Design review of the part built by this model. Coordinates are the model's own, in mm. A direction names the side the tool comes from. Give positions to 0.01 mm unless a question says otherwise; leave off trailing zeros. Loops run counter-clockwise (first coordinate to the right, second up) from the corner with the lowest first, then second, coordinate; pieces in that order, holes last. Notation, with made-up numbers: (7, 59) -> (35, 59) arc R20 cw to (35, 79) -> close; hole circle Ø3 at (24.5, 27). An arc over 180 degrees is marked (long way). Use a Markdown table: item, result. Add a question column.
1. For pin 1 Ø6 at (y, z) = (-5, 3) entering from -X; pin 2 Ø1.5 at (x, y) = (9, -1) entering from -Z; pin 3 Ø1.8 at (x, y) = (5.5, 18.5) entering from +Z; pin 4 Ø3 at (x, y) = (9, 17) entering from -Z, all flat-tipped, find the tip position at first contact; note any pin that passes through.
2. Add section D-D (z = 19). State the section outline as (x, y) points.
3. Draft analysis for pull direction X (two halves, no side actions). For faces 1 (the flat face through (0, 0, 14)), 2 (the flat face through (8, -16, 25)), 3 (the flat face through (5, -23, 32)), state which applies: pulls with the +X half, pulls with the -X half, needs draft (parallel to the pull), parting line crosses it, or undercut.
4. Add section B-B (z = 5.5). State the section outline as (x, y) points.
5. For faces 4 (the cylindrical face through (5, 0, -14)), 5 (the flat face through (5, 21, 25)), list the 3-axis set-ups (+Z, -Z, +X, -X, +Y, -Y) from which the entire face can be reached by the end or side of a thin tool; tool diameter is ignored.
6. To check wall thickness, follow line 1 (Z direction, x = 4.25, y = 0); line 2 (Y direction, x = 6.75, z = 26.5); line 3 (X direction, y = -16, z = 29.5). State the ranges of each line that lie inside material, in increasing order.
7. Add section C-C (y = -15). State the section outline as (x, z) points.
8. Add section A-A (y = 0). State the section outline as (x, z) points, and give its area (3 significant figures).
```python
from build123d import *

# Parameters (mm, degrees)
F0_R     = 10
F1_DEPTH = 10
F2_R     = 1
F3_R     = 2
F4_W     = 6
F4_H     = 10
F5_DEPTH = 15
F6_R     = 2


with BuildPart() as f1:
    # F0 (on Right) → F1 (new body)
    with BuildSketch(Plane.YZ):
        with BuildLine():
            Line((24, 32), (-24, 32))
            Line((-24, 32), (-24, 18))
            Line((-24, 18), (-14, 0))
            ThreePointArc((-14, 0), (0, -14), (14, 0))
            Line((14, 0), (24, 18))
            Line((24, 18), (24, 32))
        make_face()
        Circle(F0_R, mode=Mode.SUBTRACT)
    extrude(amount=F1_DEPTH)

    # F2
    f2_edges = [f1.edges().sort_by_distance(p)[0] for p in [
        (0, 0, -14),
        (10, 0, -14),
    ]]
    fillet(f2_edges, radius=F2_R)

    # F3
    f3_edges = [f1.edges().sort_by_distance(p)[0] for p in [
        (0, 0, 32),
        (10, 0, 32),
    ]]
    fillet(f3_edges, radius=F3_R)

    # F4 (on face) → F5 (cut)
    with BuildSketch(Plane.XY.offset(32)):
        with Locations((5, 16)):
            Rectangle(F4_W, F4_H)
        with Locations((5, -16)):
            Rectangle(F4_W, F4_H)
    extrude(amount=-F5_DEPTH, mode=Mode.SUBTRACT)

    # F6
    f6_edges = [f1.edges().sort_by_distance(p)[0] for p in [
        (2, 21, 24.5),
        (8, 21, 24.5),
        (8, 11, 24.5),
        (2, 11, 24.5),
        (2, -21, 24.5),
        (8, -21, 24.5),
        (8, -11, 24.5),
        (2, -11, 24.5),
    ]]
    fillet(f6_edges, radius=F6_R)


solid = f1.part
```
Taken from the geometry:
| question | item | result |
|---|---|---|
| 1 | pin 1 | passes through |
| 1 | pin 2 | stops at z = -14 |
| 1 | pin 3 | stops at z = 17 |
| 1 | pin 4 | stops at z = 2.7 |
| 2 | outline | (0, -24) -> (10, -24) -> (10, 24) -> (0, 24) -> close; hole (2, -19) arc R2 ccw to (4, -21) -> (6, -21) arc R2 ccw to (8, -19) -> (8, -13) arc R2 ccw to (6, -11) -> (4, -11) arc R2 ccw to (2, -13) -> close; hole (2, 13) arc R2 ccw to (4, 11) -> (6, 11) arc R2 ccw to (8, 13) -> (8, 19) arc R2 ccw to (6, 21) -> (4, 21) arc R2 ccw to (2, 19) -> close |
| 3 | face 1 | pulls with the -X half |
| 3 | face 2 | undercut |
| 3 | face 3 | needs draft |
| 4 | outline | (0, -17.06) -> (10, -17.06) -> (10, -8.35) -> (0, -8.35) -> close; (0, 8.35) -> (10, 8.35) -> (10, 17.06) -> (0, 17.06) -> close |
| 5 | face 4 | -Z, +X, -X |
| 5 | face 5 | +Z |
| 6 | line 1 | z = -14 to -10, 10 to 32 |
| 6 | line 2 | y = -24 to -20.85, -11.15 to 11.15, 20.85 to 24 |
| 6 | line 3 | x = 0 to 2, 8 to 10 |
| 7 | outline | (0, 1.8) -> (10, 1.8) -> (10, 30) arc R2 ccw to (8, 32) -> (8, 17) -> (2, 17) -> (2, 32) arc R2 ccw to (0, 30) -> close |
| 8 | outline | (0, -13) arc R1 ccw to (1, -14) -> (9, -14) arc R1 ccw to (10, -13) -> (10, -10) -> (0, -10) -> close; (0, 10) -> (10, 10) -> (10, 30) arc R2 ccw to (8, 32) -> (2, 32) arc R2 ccw to (0, 30) -> close |
| 8 | area | 258 mm^2 |
